from build123d import *

# Parameters (mm, degrees)
SKETCH1_W                                     = 76.2
SKETCH1_H                                     = 25.4
BOSS_EXTRUDE1_DEPTH                           = 6.35
CSK_FOR_1_4_FLAT_HEAD_MACHINE_SCREW1_AT_COUNT = 2
CSK_FOR_1_4_FLAT_HEAD_MACHINE_SCREW1_AT_PITCH = 38.1


with BuildPart() as part:
    # Sketch1 → Boss-Extrude1 (new body)
    with BuildSketch(Plane(origin=(0, 0, 0), x_dir=(1, 0, 0), z_dir=(0, 1, 0))):
        with Locations((38.1, 12.7)):
            Rectangle(SKETCH1_W, SKETCH1_H)
    extrude(amount=-BOSS_EXTRUDE1_DEPTH)

    # Sketch3 → CSK for 1/4 Flat Head Machine Screw1 (revolve, cut)
    with BuildSketch(Plane(origin=(19.05, 0, -7.839304919), x_dir=(0, 0, 1), z_dir=(1, 0, 0))):
        Polygon((0, 0), (0, 6.35), (3.3782, 6.35), (3.3782, 4.119929414), (6.9596, 0), align=None)
    csk_for_1_4_flat_head_machine_screw1 = revolve(axis=Axis((19.05, 6.35, -7.839304919), (0, -1, 0)), mode=Mode.SUBTRACT)

    # CSK for 1/4 Flat Head Machine Screw1 at: CSK for 1/4 Flat Head Machine Screw1 ×2
    with Locations(*[(i * CSK_FOR_1_4_FLAT_HEAD_MACHINE_SCREW1_AT_PITCH, 0, 0) for i in range(1, CSK_FOR_1_4_FLAT_HEAD_MACHINE_SCREW1_AT_COUNT)]):
        add(csk_for_1_4_flat_head_machine_screw1, mode=Mode.SUBTRACT)


solid = part.part
Verification items for the finished model (mm, model axes). Give positions to 0.01 mm unless a question says otherwise; leave off trailing zeros. Write each loop counter-clockwise with the first axis right and the second up, starting at its lowest first coordinate (ties: lowest second). Pieces come first, ordered by that corner, then holes.
(1) Cross-section at B-B (y = -1.5). Enter the section's corners in (x, z).
(2) Mould release check, pull along X, two halves, no side actions. Record for faces 1 (the face through (76.2, -3, -13)), 2 (the face through (60.147, -5.219, -6.28)), 3 (the face through (38, -6.35, -13)): +X half, -X half, draft (parallel to the pull), parting line (faces both ways), or undercut.
(3) Material ranges on line 1 (X direction, y = -5.5, z = -8); line 2 (X direction, y = -3.5, z = -9); line 3 (Z direction, x = 19.05, y = -5.7), recorded low to high.
(4) Gauge pin test, flat end, axial feed: pin 1 (8 mm diameter, centred on x = 57.15, z = -7.84, fed in from +Y). Record the tip position at first contact, or that the pin passes through.
(5) Cross-section at A-A (x = 19.05). Enter the section's corners in (y, z), plus the area to 3 significant figures.
(6) Cross-section at C-C (z = -10.5). State how many separate pieces and enclosed holes the cut face has, plus the area to 3 significant figures.
Worked out:
1. outline: (0, -25.4) - (76.2, -25.4) - (76.2, 0) - (0, 0) - close; hole circle Ø11.31 at (19.05, -7.84); hole circle Ø11.31 at (57.15, -7.84)
2. face 1: +X half
2. face 2: undercut
2. face 3: draft
3. line 1: x = 0 to 15.68, 22.42 to 53.78, 60.52 to 76.2
3. line 2: x = 0 to 15.31, 22.79 to 53.41, 60.89 to 76.2
3. line 3: z = -25.4 to -11.22, -4.46 to 0
4. pin 1: stops at y = -3.4
5. outline: (-6.35, -25.4) - (0, -25.4) - (0, -14.8) - (-4.12, -11.22) - (-6.35, -11.22) - close; (-6.35, -4.46) - (-4.12, -4.46) - (0, -0.88) - (0, 0) - (-6.35, 0) - close
5. area: 104 mm2
6. separate pieces: 3
6. enclosed holes: 0
6. area: 393 mm2
